from build123d import *

# Parameters (mm, degrees)
SKETCH1_R           = 1.5
SKETCH1_R_2         = 1
BOSS_EXTRUDE1_DEPTH = 2.5
SKETCH2_R           = 1.5
SKETCH2_R_2         = 1
BOSS_EXTRUDE2_DEPTH = 1
BOSS_EXTRUDE3_DEPTH = 3
BOSS_EXTRUDE4_DEPTH = 28
BOSS_EXTRUDE5_DEPTH = 1


with BuildPart() as part:
    # Sketch1 → Boss-Extrude1 (new body)
    with BuildSketch(Plane(origin=(0, 0, 0), x_dir=(1, 0, 0), z_dir=(0, 1, 0))):
        Circle(SKETCH1_R)
        Circle(SKETCH1_R_2, mode=Mode.SUBTRACT)
    extrude(amount=BOSS_EXTRUDE1_DEPTH)

    # Sketch2 → Boss-Extrude2 (add)
    with BuildSketch(Plane(origin=(0, 2.5, 0), x_dir=(1, 0, 0), z_dir=(0, 1, 0))):
        Circle(SKETCH2_R)
        Circle(SKETCH2_R_2, mode=Mode.SUBTRACT)
        with BuildLine():
            ThreePointArc((0, 1.5), (1.060660172, 1.060660172), (1.5, 0))
            Line((1.5, 0), (1.5, 1))
            Line((1.5, 1), (1, 1.5))
            Line((1, 1.5), (0, 1.5))
        make_face()
        with BuildLine():
            ThreePointArc((1.5, 0), (1.060660172, -1.060660172), (0, -1.5))
            Line((0, -1.5), (1.3, -1.5))
            Line((1.3, -1.5), (1.5, -1.5))
            Line((1.5, -1.5), (1.5, 0))
        make_face()
        with BuildLine():
            Line((-1.3, -1.5), (0, -1.5))
            ThreePointArc((0, -1.5), (-1.060660172, -1.060660172), (-1.5, 0))
            Line((-1.5, 0), (-1.5, -1.5))
            Line((-1.5, -1.5), (-1.3, -1.5))
        make_face()
        with BuildLine():
            Line((-1.5, 1), (-1.5, 0))
            ThreePointArc((-1.5, 0), (-1.060660172, 1.060660172), (0, 1.5))
            Line((0, 1.5), (-1, 1.5))
            Line((-1, 1.5), (-1.5, 1))
        make_face()
        Polygon((1.3, -1.5), (0, -1.5), (-1.3, -1.5), (-1.3, -3), (-0.8, -3), (0.8, -3), (1.3, -3), align=None)
        Polygon((0.8, -3), (-0.8, -3), (-0.8, -3.5), (-0.8, -5.5), (0.8, -5.5), (0.8, -3.5), align=None)
        Polygon((-0.8, -3), (-1.3, -3), (-0.8, -3.5), align=None)
        Polygon((0.8, -3.5), (1.3, -3), (0.8, -3), align=None)
    extrude(amount=-BOSS_EXTRUDE2_DEPTH)

    # Sketch3 → Boss-Extrude3 (add)
    with BuildSketch(Plane.XY.offset(5.5)):
        with BuildLine():
            ThreePointArc((-0.4, 2), (0, 2.4), (0.4, 2))
            Line((0.4, 2), (0.5, 2))
            ThreePointArc((0.5, 2), (0.353553391, 2.353553391), (0, 2.5))
            ThreePointArc((0, 2.5), (-0.353553391, 2.353553391), (-0.5, 2))
            Line((-0.5, 2), (-0.4, 2))
        make_face()
        with BuildLine():
            Line((0.5, 2), (0.4, 2))
            ThreePointArc((0.4, 2), (0, 1.6), (-0.4, 2))
            Line((-0.4, 2), (-0.5, 2))
            ThreePointArc((-0.5, 2), (-0.353553391, 1.646446609), (0, 1.5))
            ThreePointArc((0, 1.5), (0.353553391, 1.646446609), (0.5, 2))
        make_face()
    extrude(amount=BOSS_EXTRUDE3_DEPTH)

    # Sketch3_3 → Boss-Extrude4 (add)
    with BuildSketch(Plane.XY.offset(5.5)):
        with BuildLine():
            ThreePointArc((-0.4, 2), (0, 1.6), (0.4, 2))
            Line((0.4, 2), (-0.4, 2))
        make_face()
        with BuildLine():
            Line((-0.4, 2), (0.4, 2))
            ThreePointArc((0.4, 2), (0, 2.4), (-0.4, 2))
        make_face()
    extrude(amount=BOSS_EXTRUDE4_DEPTH)

    # Sketch4 → Boss-Extrude5 (add)
    with BuildSketch(Plane(origin=(0, 2.5, 0), x_dir=(1, 0, 0), z_dir=(0, 1, 0))):
        Polygon((1.3, -1.5), (1.5, -1.5), (1.5, 1), (1, 1.5), (-1, 1.5), (-1.5, 1), (-1.5, -1.5), (-1.3, -1.5), (-1.3, -3), (-0.8, -3.5), (-0.8, -5.5), (0, -5.5), (0.8, -5.5), (0.8, -3.5), (1.3, -3), align=None)
    extrude(amount=-BOSS_EXTRUDE5_DEPTH)


solid = part.part
Could you check a few things on this model? Use its own coordinates, in mm. A direction names the side the tool comes from. Coordinates: 2 decimals unless noted, no trailing zeros. Order: outer loops, then holes, each group sorted by start corner. A loop starts at its lowest first (then second) coordinate and runs counter-clockwise, first axis right, second up. Notation, with made-up numbers: (-4, -26.75) - (44, -26.75) arc R13 cw to (44, -10.75) - close; hole circle Ø9 at (41, 67.25). An arc over 180 degrees is marked (long way). Answer in a Markdown table with one row per item. Add a question column.
(1) If we section it at C-C, the plane z = 23: Please give me the cut outline in (x, y).
(2) On a 3-axis mill with a long thin cutter (end or side, diameter ignored), from which of +Z, -Z, +X, -X, +Y, -Y can I reach the whole of each face in a straight line? I mean faces 1 (the face through (0.8, 2, 5)), 2 (the face through (1.5, 2, 0)), 3 (the face through (-0.8, 2, 4)). Say none if no direction works.
(3) Will these pins go through, and if not, where does the flat tip stop? pin 1 (1.5 mm diameter, centred on x = 0.5, z = 29, fed in from -Y); pin 2 (0.8 mm diameter, centred on y = 2, z = 4, fed in from +X); pin 3 (1.5 mm diameter, centred on y = 1, z = 24.5, fed in from -X).
(4) If we mould it in two halves opening along X, with no side actions, what happens to faces 4 (the face through (0, 1.5, 0)), 5 (the face through (0, 1, 1)), 6 (the face through (-1.5, 0.74, -0.07)), 7 (the face through (0, 2, -1.5))? For each: released by +X, released by -X, zero draft, split by the parting line, or undercut.
(5) If we section it at A-A, the plane y = 1.05: Please give me the cut outline in (x, z), then the cut area to 3 significant figures.
(6) I need wall thicknesses on L1, parallel to Z at x = -0.1, y = 0.7; L2, parallel to X at y = 0.75, z = 0; L3, parallel to Z at x = 0.35, y = 0.45. Which ranges of each line are inside material? Lowest first, please.
(7) If we section it at B-B, the plane z = 5: Please give me the cut outline in (x, y), then the cut area to 3 significant figures.
Results are:
| question | item | result |
|---|---|---|
| 1 | outline | circle Ø0.8 at (0, 2) |
| 2 | face 1 | +Z, +X, +Y, -Y |
| 2 | face 2 | +Z, -Z, +X, +Y, -Y |
| 2 | face 3 | +Z, -X, +Y, -Y |
| 3 | pin 1 | stops at y = 1.6 |
| 3 | pin 2 | stops at x = 0.8 |
| 3 | pin 3 | stops at x = -0.31 |
| 4 | face 4 | undercut |
| 4 | face 5 | undercut |
| 4 | face 6 | split by the parting line |
| 4 | face 7 | zero draft |
| 5 | outline | circle Ø3 at (0, 0); hole circle Ø2 at (0, 0) |
| 5 | area | 3.93 mm2 |
| 6 | L1 | z = -1.5 to -0.99, 0.99 to 1.5 |
| 6 | L2 | x = -1.5 to -1, 1 to 1.5 |
| 6 | L3 | z = -1.46 to -0.94, 0.94 to 1.46 |
| 7 | outline | (-0.8, 1.5) - (0.8, 1.5) - (0.8, 2.5) - (-0.8, 2.5) - close |
| 7 | area | 1.60 mm2 |
